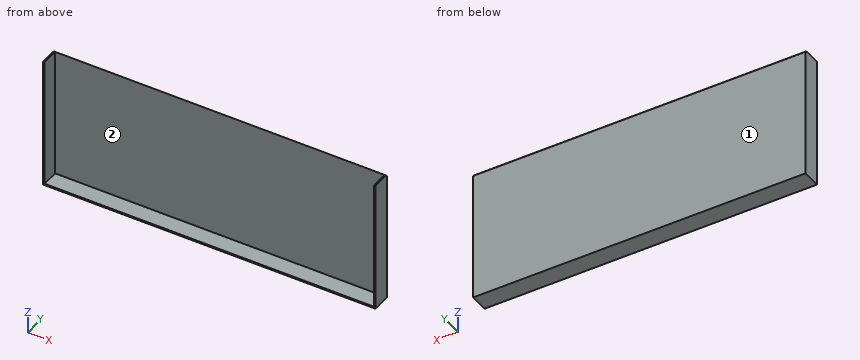
```python
from build123d import *

# Parameters (mm, degrees)
DODANIE_WYCI_GNI_CIE3_DEPTH = 193.5
DODANIE_WYCI_GNI_CIE4_DEPTH = 20


with BuildPart() as part:
    # Szkic3 → Dodanie-wyciągnięcie3 (new body, symmetric)
    with BuildSketch(Plane(origin=(0, 0, 0), x_dir=(0, 0, -1), z_dir=(1, 0, 0))):
        Polygon((0, 0), (-150, 0), (-151.75, -1.75), (0, -1.75), align=None)
    extrude(amount=DODANIE_WYCI_GNI_CIE3_DEPTH, both=True)

    # Szkic4 → Dodanie-wyciągnięcie4 (add)
    with BuildSketch(Plane.XZ.offset(1.75)):
        Polygon((-193.5, 151.75), (-193.5, 0), (193.5, 0), (193.5, 151.75), (191.75, 151.75), (191.75, 1.75), (-191.75, 1.75), (-191.75, 151.75), align=None)
    extrude(amount=DODANIE_WYCI_GNI_CIE4_DEPTH)


solid = part.part
```
CAD build for the part. Positions are in the model's coordinates, mm. Face numbers are marked on the shaded views. Coordinates: 2 decimals unless noted, no trailing zeros. Loops run counter-clockwise (first coordinate to the right, second up) from the corner with the lowest first, then second, coordinate; pieces in that order, holes last. Notation, with made-up numbers: (62.25, 78) - (110.25, 78) arc R18 ccw to (110.25, 108) - close; hole circle Ø10 at (-36.75, -32.5). An arc over 180 degrees is marked (long way). Return JSON: item names as keys, results as strings.
1. Probe L1, parallel to X at y = -8, z = 22; L2, parallel to Z at x = -144.5, y = -9; L3, parallel to Y at x = 166.5, z = 144.5. List the from-to ranges inside material, lowest first. Write a range as from..to.
Result:
{"L1": "x = -193.5..-191.75, 191.75..193.5", "L2": "z = 0..1.75", "L3": "y = -1.75..0"}
2. Band-saw the part on C-C (x = 168). Give the cut face in (y, z), and give its area (3 significant figures).
Result:
{"outline": "(-21.75, 0) - (0, 0) - (0, 150) - (-1.75, 151.75) - (-1.75, 1.75) - (-21.75, 1.75) - close", "area": "299 mm2"}
3. Drop flat-ended pins along their axis: pin 1 (10 mm diameter, centred on x = 34.5, y = -13.5, fed in from +Z); pin 2 (3 mm diameter, centred on x = -55, z = 52.5, fed in from +Y); pin 3 (1 mm diameter, centred on x = -45.5, z = 78.5, fed in from -Y). Give the stop position or say it passes through.
Result:
{"pin 1": "stops at z = 1.75", "pin 2": "stops at y = 0", "pin 3": "stops at y = -1.75"}
4. Band-saw the part on B-B (z = 141.5). Give the cut face in (x, y).
Result:
{"outline": "(-193.5, -21.75) - (-191.75, -21.75) - (-191.75, -1.75) - (191.75, -1.75) - (191.75, -21.75) - (193.5, -21.75) - (193.5, 0) - (-193.5, 0) - close"}
5. Band-saw the part on A-A (y = -8). Give the cut face in (x, z).
Result:
{"outline": "(-193.5, 0) - (193.5, 0) - (193.5, 151.75) - (191.75, 151.75) - (191.75, 1.75) - (-191.75, 1.75) - (-191.75, 151.75) - (-193.5, 151.75) - close"}
6. Mould opens along X. For the marked faces 1 and 2 say: released by +X, released by -X, zero draft, split by the parting line, or undercut.
Result:
{"face 1": "zero draft", "face 2": "undercut"}
